The listing builds one solid part. Answer for the finished solid, in the listing's coordinates (mm). A direction names the side the tool comes from. Give positions to 0.01 mm unless a question says otherwise; leave off trailing zeros. Loops run counter-clockwise (first coordinate to the right, second up) from the corner with the lowest first, then second, coordinate; pieces in that order, holes last.
Item 1: Consider line 1 along Z through (x, y) = (6.25, 1.5); line 2 along Y through (x, z) = (-4.5, 3.5); line 3 along Y through (x, z) = (3.25, 4.55). Determine where each line is inside the solid, lowest interval first.
Item 2: Section C-C, the plane x = -4.5 is taken. Give the vertices of the cut face in (y, z), and give its area (3 significant figures).
Item 3: Section A-A, the plane x = 6.25 is taken. Give the vertices of the cut face in (y, z), and give its area (3 significant figures).
Item 4: A tool of negligible diameter and unlimited length cuts with its end or side. For faces 1 (the face through (0, 8, 3)), 2 (the face through (0, -5, 4)), 3 (the face through (-6, 1, 3)), 4 (the face through (6, 1, 3)), from which of +Z, -Z, +X, -X, +Y, -Y can it reach the whole face along a straight path? Write none if from no direction.
Item 5: Section B-B, the plane y = 6.25 is taken. Give the vertices of the cut face in (x, z), and give its area (3 significant figures).
Item 6: Each of these flat-tipped pins is pushed along its axis until it touches: pin 1 Ø1 at (x, z) = (-5, 5) entering from -Y; pin 2 Ø1 at (x, y) = (1.5, 7) entering from +Z; pin 3 Ø2 at (x, z) = (-1.5, 4.5) entering from +Y. Where does it stop, or does it pass through?
Item 7: The mould has two halves that part along Z. Classify faces 5 (the face through (0, 1, 6)), 6 (the face through (0, 0, 0)), 7 (the face through (-7, 1, 4)), 8 (the face through (0, 6, 5)): pulls with the +Z half, pulls with the -Z half, needs draft (parallel to the pull), parting line crosses it, or undercut.
Item 8: Section D-D, the plane z = 2.8 is taken. Give the vertices of the cut face in (x, y).
from build123d import *

# Parameters (mm, degrees)
F1_W     = 16
F1_H     = 20
F2_DEPTH = 2
F3_W     = 12
F3_H     = 14
F4_DEPTH = 2
F5_W     = 2
F5_H     = 10
F5_W_2   = 12
F6_DEPTH = 2


with BuildPart() as f2:
    # F1 (on Top) → F2 (new body)
    with BuildSketch(Plane.XY):
        Rectangle(F1_W, F1_H)
    extrude(amount=F2_DEPTH)

    # F3 (on face) → F4 (join)
    with BuildSketch(Plane.XY.offset(2)):
        with Locations((0, 1)):
            Rectangle(F3_W, F3_H)
    extrude(amount=F4_DEPTH)

    # F5 (on face) → F6 (join)
    with BuildSketch(Plane.XY.offset(4)):
        with Locations((-7, 1)):
            Rectangle(F5_W, F5_H)
        with Locations((0, 1)):
            Rectangle(F5_W_2, F5_H)
        with Locations((7, 1)):
            Rectangle(F5_W, F5_H)
    extrude(amount=F6_DEPTH)


solid = f2.part
Worked answers:
1. line 1: z = 0 to 2, 4 to 6
1. line 2: y = -6 to 8
1. line 3: y = -4 to 6
2. outline: (-10, 0) - (10, 0) - (10, 2) - (8, 2) - (8, 4) - (6, 4) - (6, 6) - (-4, 6) - (-4, 4) - (-6, 4) - (-6, 2) - (-10, 2) - close
2. area: 88.0 mm2
3. outline: (-10, 0) - (10, 0) - (10, 2) - (-10, 2) - close; (-4, 4) - (6, 4) - (6, 6) - (-4, 6) - close
3. area: 60.0 mm2
4. face 1: +Z, +X, -X, +Y
4. face 2: +Z, +X, -X, -Y
4. face 3: -X, +Y, -Y
4. face 4: +X, +Y, -Y
5. outline: (-8, 0) - (8, 0) - (8, 2) - (6, 2) - (6, 4) - (-6, 4) - (-6, 2) - (-8, 2) - close
5. area: 56.0 mm2
6. pin 1: stops at y = -4
6. pin 2: stops at z = 4
6. pin 3: stops at y = 8
7. face 5: pulls with the +Z half
7. face 6: pulls with the -Z half
7. face 7: undercut
7. face 8: needs draft
8. outline: (-6, -6) - (6, -6) - (6, 8) - (-6, 8) - close
